Here's how the part is built. I have some questions about the finished solid (model axes, mm). A direction names the side the tool comes from. Coordinates: 2 decimals unless noted, no trailing zeros. Write each loop counter-clockwise with the first axis right and the second up, starting at its lowest first coordinate (ties: lowest second). Pieces come first, ordered by that corner, then holes. Notation, with made-up numbers: M 20.5,7 L 25.5,7 A22 ccw 25.5,33 Z; hole C 16.25,32 d10. An arc over 180 degrees is marked long. Use a Markdown table: item, result.
```python
from build123d import *

# Parameters (mm, degrees)
F1_DEPTH = 15
F2_DEPTH = 2


with BuildPart() as f1:
    # F0 (on Right) → F1 (new body)
    with BuildSketch(Plane.YZ):
        with BuildLine():
            Line((-18.500151, -15.885202), (21.499849, -15.885202))
            ThreePointArc((21.499849, -15.885202), (28.776178, 4.748888), (18.594223, 24.114798))
            Line((18.594223, 24.114798), (-1.211139, 21.331336))
            ThreePointArc((-1.211139, 21.331336), (-5.644923, 17.678725), (-10.913745, 19.967723))
            Line((-10.913745, 19.967723), (-20.816425, 18.575992))
            ThreePointArc((-20.816425, 18.575992), (-25.786783, 0.933475), (-18.500151, -15.885202))
        make_face()
        with BuildLine():
            ThreePointArc((-18.016041, -14.785202), (-24.689377, 1.008996), (-20.187486, 17.553574))
            Line((-20.187486, 17.553574), (-11.387244, 18.790367))
            ThreePointArc((-11.387244, 18.790367), (-5.491832, 16.589431), (-0.431459, 20.330102))
            Line((-0.431459, 20.330102), (18.271464, 22.958627))
            ThreePointArc((18.271464, 22.958627), (27.678942, 4.670945), (21.015738, -14.785202))
            Line((21.015738, -14.785202), (-18.016041, -14.785202))
        make_face(mode=Mode.SUBTRACT)
    extrude(amount=F1_DEPTH)

    # F0 (on Right) → F2 (join)
    with BuildSketch(Plane.YZ):
        with BuildLine():
            Line((-11.387244, 18.790367), (-20.187486, 17.553574))
            ThreePointArc((-20.187486, 17.553574), (-24.689377, 1.008996), (-18.016041, -14.785202))
            Line((-18.016041, -14.785202), (21.015738, -14.785202))
            ThreePointArc((21.015738, -14.785202), (27.678942, 4.670945), (18.271464, 22.958627))
            Line((18.271464, 22.958627), (-0.431459, 20.330102))
            ThreePointArc((-0.431459, 20.330102), (-5.491832, 16.589431), (-11.387244, 18.790367))
        make_face()
    extrude(amount=F2_DEPTH)


solid = f1.part
```
1. Which directions (+Z, -Z, +X, -X, +Y, -Y) give clear straight access to the entire face, cutting with the end or side of a thin tool? Please do faces 4 (the face through (7.4, -5.56, 17.69)), 5 (the face through (8.409, -15.849, 18.163)).
Answers follow:
| item | result |
|---|---|
| face 4 | +Z, +X, -X |
| face 5 | +X |
2. Will these pins go through, and if not, where does the flat tip stop? pin 1 Ø1 at (x, z) = (12.5, 1) entering from +Y; pin 2 Ø5 at (x, z) = (9.5, 7.5) entering from -Y; pin 3 Ø8 at (x, y) = (10, 6) entering from +Z.
Answers follow:
| item | result |
|---|---|
| pin 1 | stops at y = 28.82 |
| pin 2 | stops at y = -25.76 |
| pin 3 | stops at z = 22.91 |
3. I need wall thicknesses on probe 1 along X at (y, z) = (2, 14); probe 2 along Y at (x, z) = (14.25, -9); probe 3 along Y at (x, z) = (10, 4.5). Which ranges of each line are inside material? Lowest first, please.
Answers follow:
| item | result |
|---|---|
| probe 1 | x = 0 to 2 |
| probe 2 | y = -23.19 to -21.96, 24.96 to 26.19 |
| probe 3 | y = -25.79 to -24.69, 27.69 to 28.79 |
4. Suppose I cut it at A-A on x = 6.75. Write out the boundary of the cut face in (y, z), and give its area (3 significant figures).
Answers follow:
| item | result |
|---|---|
| outline | M -20.82,18.58 A27.35 ccw -18.5,-15.89 L 21.5,-15.89 A27.35 ccw 18.59,24.11 L -1.21,21.33 A5.5 cw -10.91,19.97 Z; hole M -20.19,17.55 A26.25 ccw -18.02,-14.79 L 21.02,-14.79 A26.25 ccw 18.27,22.96 L -0.43,20.33 A6.6 cw -11.39,18.79 Z |
| area | 177 mm2 |
5. We'd pull the mould along Y, two halves only. Please class faces 1 (the face through (7.395, 8.83, 22.743)), 2 (the face through (7, 1, -15.885)), 3 (the face through (8.409, 8.789, 21.626)): +Y half, -Y half, draft (parallel to the pull), parting line (faces both ways), or undercut.
Answers follow:
| item | result |
|---|---|
| face 1 | -Y half |
| face 2 | draft |
| face 3 | undercut |
6. Suppose I cut it at C-C on y = -2. Write out the boundary of the cut face in (x, z), and give its area (3 significant figures).
Answers follow:
| item | result |
|---|---|
| outline | M 0,-15.89 L 15,-15.89 L 15,-14.79 L 2,-14.79 L 2,18.22 L 15,18.22 L 15,19.84 L 0,19.84 Z |
| area | 107 mm2 |
7. Suppose I cut it at B-B on z = -7. Write out the boundary of the cut face in (x, y).
Answers follow:
| item | result |
|---|---|
| outline | M 0,-24.04 L 15,-24.04 L 15,-22.86 L 2,-22.86 L 2,25.86 L 15,25.86 L 15,27.04 L 0,27.04 Z |
